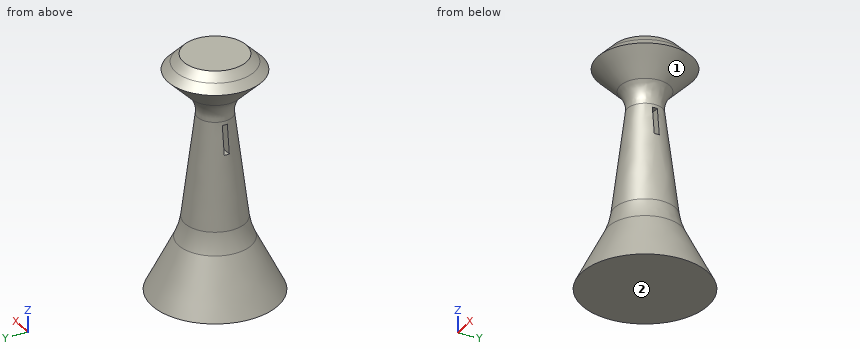
```python
from build123d import *

# Parameters (mm, degrees)
F0_R           = 12.7
F2_R           = 6.35
F3_FACE_R      = 6.35
F5_R           = 3.175
F6_FACE_R      = 3.175
F8_R           = 9.525
F10_R          = 12.7
F11_R          = 5.08
F9_FACE_R      = 9.525
F13_R          = 7.9375
F16_R          = 6.35
F14_FACE_R     = 7.9375
F18_W          = 0.508
F18_H          = 5.6896
F19_DEPTH      = 12.7010001
F19_DEPTH_BACK = 25.4
F20_DEPTH      = 1.27


with BuildPart() as f3:
    # F0 (on Top) → F3 section 0
    with BuildSketch(Plane.XY):
        Circle(F0_R)
    # F2 (on offset) → F3 section 1
    with BuildSketch(Plane.XY.offset(12.7)):
        Circle(F2_R)
    loft()

    # F3_face (on face) → F6 section 0
    with BuildSketch(Plane.XY.offset(12.7)):
        Circle(F3_FACE_R)
    # F5 (on offset) → F6 section 1
    with BuildSketch(Plane.XY.offset(38.1)):
        Circle(F5_R)
    loft()

    # F6_face (on face) → F9 section 0
    with BuildSketch(Plane.XY.offset(38.1)):
        Circle(F6_FACE_R)
    # F8 (on offset) → F9 section 1
    with BuildSketch(Plane.XY.offset(44.45)):
        Circle(F8_R)
    loft()

    # F10
    f10_edges = [f3.edges().sort_by_distance(p)[0] for p in [
        (-6.35, 0, 12.7),
    ]]
    fillet(f10_edges, radius=F10_R)

    # F11
    f11_edges = [f3.edges().sort_by_distance(p)[0] for p in [
        (-3.175, 0, 38.1),
    ]]
    fillet(f11_edges, radius=F11_R)

    # F9_face (on face) → F14 section 0
    with BuildSketch(Plane.XY.offset(44.45)):
        Circle(F9_FACE_R)
    # F13 (on offset) → F14 section 1
    with BuildSketch(Plane.XY.offset(46.0375)):
        Circle(F13_R)
    loft()

    # F16 (on offset) → F17 section 0
    with BuildSketch(Plane.XY.offset(47.625)):
        Circle(F16_R)
    # F14_face (on face) → F17 section 1
    with BuildSketch(Plane.XY.offset(46.0375)):
        Circle(F14_FACE_R)
    loft()

    # F18 (on Right) → F19 (cut, two sides)
    with BuildSketch(Plane.YZ) as f19_sk:
        with Locations((0.254, 32.0802)):
            Rectangle(F18_W, F18_H)
        with Locations((-0.254, 32.0802)):
            Rectangle(F18_W, F18_H)
    extrude(amount=-F19_DEPTH, mode=Mode.SUBTRACT)
    extrude(f19_sk.sketch, amount=F19_DEPTH_BACK, mode=Mode.SUBTRACT)

    # F18 (on Right) → F20 (join, symmetric)
    with BuildSketch(Plane.YZ):
        with Locations((0.254, 32.0802)):
            Rectangle(F18_W, F18_H)
        with Locations((-0.254, 32.0802)):
            Rectangle(F18_W, F18_H)
    extrude(amount=F20_DEPTH, both=True)


solid = f3.part
```
Could you check a few things on this model? Use its own coordinates, in mm. Face numbers are marked on the shaded views. A direction names the side the tool comes from. Give positions to 0.01 mm unless a question says otherwise; leave off trailing zeros. Write each loop counter-clockwise with the first axis right and the second up, starting at its lowest first coordinate (ties: lowest second). Pieces come first, ordered by that corner, then holes. Notation, with made-up numbers: (-11, 60) -> (22, 60) arc R26 cw to (22, 86) -> close; hole circle Ø2 at (-26, 80.5). An arc over 180 degrees is marked (long way). Write each question's results on one line, items separated by ' | '.
1. Will these pins go through, and if not, where does the flat tip stop? pin 1 Ø10 at (y, z) = (-9, 28) entering from +X; pin 2 Ø4 at (x, z) = (-6.5, 18) entering from +Y; pin 3 Ø0.9 at (x, z) = (2, 31.5) entering from -Y.
Check sheet entries:
pin 1: stops at x = 2.02 | pin 2: stops at y = 3.51 | pin 3: stops at y = -3.7
2. On a 3-axis mill with a long thin cutter (end or side, diameter ignored), from which of +Z, -Z, +X, -X, +Y, -Y can I reach the whole of each face in a straight line? I mean the marked faces 1 and 2. Say none if no direction works.
Check sheet entries:
face 1: none | face 2: -Z, +X, -X, +Y, -Y
3. I want a section at C-C, the plane z = 28.5. Write out the boundary of the cut face in (x, y) (3 decimals), then the cut area to 3 significant figures.
Check sheet entries:
outline: circle Ø8.75 at (0, 0) | area: 60.1 mm²
4. I want a section at B-B, the plane z = 6.5. Write out the boundary of the cut face in (x, y).
Check sheet entries:
outline: circle Ø18.9 at (0, 0)
5. I need wall thicknesses on L1, parallel to Z at x = -2.75, y = 0.25 (3 decimals); L2, parallel to Z at x = 6, y = 7; L3, parallel to X at y = -2, z = 8. Which ranges of each line are inside material? Lowest first, please.
Check sheet entries:
L1: z = 0 to 29.235, 34.925 to 47.625 | L2: z = 0 to 6.96, 44.14 to 44.76 | L3: x = -8.47 to 8.47
